```python
from build123d import *

# Parameters (mm, degrees)
SKETCH_1_W          = 28
SKETCH_1_H          = 8
SKETCH_1_R          = 1.525
EXTRUDE_1_DEPTH     = 1
SKETCH_2_R          = 1.525
CUT_EXTRUDE_1_DEPTH = 1
FILLET_1_R          = 2
SKETCH_3_R          = 1.525
CUT_EXTRUDE_2_DEPTH = 10
SKETCH_4_R          = 1.525
CUT_EXTRUDE_3_DEPTH = 10
EXTRUDE_2_DEPTH     = 1
FILLET_2_R          = 2


with BuildPart() as part:
    # 草图1 → 凸台-拉伸1 (new body)
    with BuildSketch(Plane.XY):
        Polygon((-4, 4), (24, 4), (42.5, 4), (42.5, 58.5), (-45, 58.5), (-45, 4), align=None)
        with Locations((10, 0)):
            Rectangle(SKETCH_1_W, SKETCH_1_H)
        with Locations((20, 0)):
            Circle(SKETCH_1_R, mode=Mode.SUBTRACT)
        Circle(SKETCH_1_R, mode=Mode.SUBTRACT)
    extrude(amount=EXTRUDE_1_DEPTH)

    # 草图2 → 切除-拉伸1 (cut)
    with BuildSketch(Plane.XY.offset(1)):
        with Locations((-40, 37.25)):
            Circle(SKETCH_2_R)
        with Locations((-40, 17.25)):
            Circle(SKETCH_2_R)
    extrude(amount=-CUT_EXTRUDE_1_DEPTH, mode=Mode.SUBTRACT)

    # 圆角1
    fillet_1_edges = [part.edges().sort_by_distance(p)[0] for p in [
        (42.5, 4, 0.5),
        (24, 4, 0.5),
        (24, -4, 0.5),
        (-4, -4, 0.5),
        (-4, 4, 0.5),
        (-45, 4, 0.5),
        (-45, 58.5, 0.5),
        (42.5, 58.5, 0.5),
    ]]
    fillet(fillet_1_edges, radius=FILLET_1_R)

    # 草图3 → 切除-拉伸2 (cut)
    with BuildSketch(Plane.XY.offset(1)):
        with Locations((39, 47.25)):
            Circle(SKETCH_3_R)
        with Locations((39, 27.25)):
            Circle(SKETCH_3_R)
    extrude(amount=-CUT_EXTRUDE_2_DEPTH, mode=Mode.SUBTRACT)

    # 草图4 → 切除-拉伸3 (cut)
    with BuildSketch(Plane.XY.offset(1)):
        with Locations((-20, 55.5)):
            Circle(SKETCH_4_R)
        with Locations((0, 55.5)):
            Circle(SKETCH_4_R)
    extrude(amount=-CUT_EXTRUDE_3_DEPTH, mode=Mode.SUBTRACT)

    # 草图5 → 凸台-拉伸2 (add)
    with BuildSketch(Plane.XY.offset(1)):
        with BuildLine():
            ThreePointArc((-45, 56.5), (-44.414213562, 57.914213562), (-43, 58.5))
            Line((-43, 58.5), (-91, 58.5))
            Line((-91, 58.5), (-105.603230987, 4))
            Line((-105.603230987, 4), (-43, 4))
            ThreePointArc((-43, 4), (-44.414213562, 4.585786438), (-45, 6))
            Line((-45, 6), (-45, 56.5))
        make_face()
    extrude(amount=-EXTRUDE_2_DEPTH)

    # 圆角2
    fillet_2_edges = [part.edges().sort_by_distance(p)[0] for p in [
        (-91, 58.5, 0.5),
        (-105.603230987, 4, 0.5),
    ]]
    fillet(fillet_2_edges, radius=FILLET_2_R)


solid = part.part
```
CAD build for the part. Positions are in the model's coordinates, mm. Round coordinates to 2 decimals unless told otherwise and drop trailing zeros. Order: outer loops, then holes, each group sorted by start corner. A loop starts at its lowest first (then second) coordinate and runs counter-clockwise, first axis right, second up. Notation, with made-up numbers: (-37, -38) -> (-24, -38) arc R26 cw to (-24, -24) -> close; hole circle Ø3 at (54, 10). An arc over 180 degrees is marked (long way). Write item = value, one per line.
(1) Cut at C-C (z = 0.25). State how many separate pieces and enclosed holes the cut face has, plus the area to 3 significant figures.
Answers follow:
separate_pieces = 1
enclosed_holes = 8
area = 7,840 mm²
(2) Cut at D-D (x = 20). Write the cut outline in (y, z) (3 decimals), plus the area to 4 significant figures.
Answers follow:
outline = (-4, 0) -> (-1.525, 0) -> (-1.525, 1) -> (-4, 1) -> close; (1.525, 0) -> (58.5, 0) -> (58.5, 1) -> (1.525, 1) -> close
area = 59.45 mm²
(3) Flat gauge pins, fed straight in: P1, Ø2.5, axis at x = 39, y = 27.25, coming from the +Z side; P2, Ø0.5, axis at x = -34.5, z = 0.5, coming from the -Y side; P3, Ø0.5, axis at y = 0, z = 0.5, coming from the +X side. Where does each tip first touch, or does it go through?
Answers follow:
P1 = through
P2 = 4
P3 = 24
(4) Drill centre lines: L1, parallel to Y at x = -40, z = 0.3 (3 decimals); L2, parallel to Y at x = 39, z = 0.75 (3 decimals); L3, parallel to X at y = 0.5, z = 0.8. Where is each one in solid material? Low to high.
Answers follow:
L1 = 4 to 15.725, 18.775 to 35.725, 38.775 to 58.5
L2 = 4 to 25.725, 28.775 to 45.725, 48.775 to 58.5
L3 = -4 to -1.44, 1.44 to 18.56, 21.44 to 24
(5) Cut at A-A (x = 39). Write the cut outline in (y, z) (3 decimals), plus the area to 3 significant figures.
Answers follow:
outline = (4, 0) -> (25.725, 0) -> (25.725, 1) -> (4, 1) -> close; (28.775, 0) -> (45.725, 0) -> (45.725, 1) -> (28.775, 1) -> close; (48.775, 0) -> (58.5, 0) -> (58.5, 1) -> (48.775, 1) -> close
area = 48.4 mm²
(6) Pull direction Y, two halves, no side cores. Call faces 1 (the flat face through (-32, 28, 1)), 2 (the cylindrical face through (-41.21, 36.32, 0.51)), 3 (the flat face through (-98.07, 32.12, 0.51)): +Y half, -Y half, draft (parallel to the pull), parting line (faces both ways), or undercut.
Answers follow:
face_1 = draft
face_2 = undercut
face_3 = +Y half
(7) Cut at B-B (y = 27.25). Write the cut outline in (x, z) (3 decimals), plus the area to 3 significant figures.
Answers follow:
outline = (-99.373, 0) -> (37.475, 0) -> (37.475, 1) -> (-99.373, 1) -> close; (40.525, 0) -> (42.5, 0) -> (42.5, 1) -> (40.525, 1) -> close
area = 139 mm²
